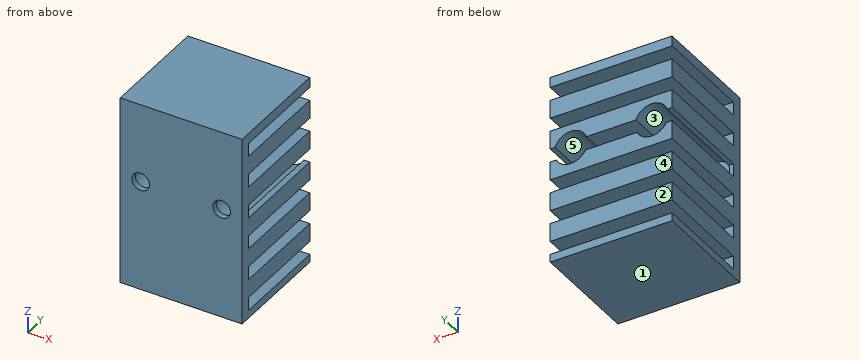
```python
from build123d import *

# Parameters (mm, degrees)
SKETCH1_W           = 11
SKETCH1_H           = 17.14
SKETCH1_R           = 0.8
BOSS_EXTRUDE1_DEPTH = 10
SKETCH3_W           = 1.2
SKETCH3_H           = 9.077755084
CUT_EXTRUDE1_DEPTH  = 18.159396843
SKETCH4_R           = 1.5
CUT_EXTRUDE2_DEPTH  = 9.5


with BuildPart() as part:
    # Sketch1 → Boss-Extrude1 (new body)
    with BuildSketch(Plane(origin=(0, 0, 0), x_dir=(1, 0, 0), z_dir=(0, 1, 0))):
        Rectangle(SKETCH1_W, SKETCH1_H)
        with Locations(Location((3.65, -1.43, 0), (0, 0, 270))):
            Circle(SKETCH1_R, mode=Mode.SUBTRACT)
        with Locations(Location((-3.65, -1.43, 0), (0, 0, 270))):
            Circle(SKETCH1_R, mode=Mode.SUBTRACT)
    extrude(amount=BOSS_EXTRUDE1_DEPTH)

    # Sketch3 → Cut-Extrude1 (cut, through all)
    with BuildSketch(Plane(origin=(5.5, 0, 0), x_dir=(0, 0, -1), z_dir=(1, 0, 0))):
        with Locations((-4.19, 5.461122458)):
            Rectangle(SKETCH3_W, SKETCH3_H)
        with Locations((-7.05, 5.461122458)):
            Rectangle(SKETCH3_W, SKETCH3_H)
        with Locations((-1.33, 5.461122458)):
            Rectangle(SKETCH3_W, SKETCH3_H)
        with Locations((1.53, 5.461122458)):
            Rectangle(SKETCH3_W, SKETCH3_H)
        with Locations((4.39, 5.461122458)):
            Rectangle(SKETCH3_W, SKETCH3_H)
        with Locations((7.25, 5.461122458)):
            Rectangle(SKETCH3_W, SKETCH3_H)
    extrude(amount=-CUT_EXTRUDE1_DEPTH, mode=Mode.SUBTRACT)

    # Sketch4 → Cut-Extrude2 (cut)
    with BuildSketch(Plane(origin=(0, 10, 0), x_dir=(1, 0, 0), z_dir=(0, 1, 0))):
        with Locations(Location((-3.65, -1.43, 0), (0, 0, 270))):
            Circle(SKETCH4_R)
        with Locations(Location((3.65, -1.43, 0), (0, 0, 270))):
            Circle(SKETCH4_R)
    extrude(amount=-CUT_EXTRUDE2_DEPTH, mode=Mode.SUBTRACT)


solid = part.part
```
Check sheet for the modelled part. Datum: model origin and axes. Units: mm. Face numbers are marked on the shaded views. A direction names the side the tool comes from. Give positions to 0.01 mm unless a question says otherwise; leave off trailing zeros. Loops run counter-clockwise (first coordinate to the right, second up) from the corner with the lowest first, then second, coordinate; pieces in that order, holes last. Notation, with made-up numbers: M 58,89 L 114,89 A21 cw 114,95 Z; hole C 6,60 d6. An arc over 180 degrees is marked long. Answer as CSV lines item,"result".
Item 1: Sectioned sample at D-D, the plane z = -7. Enter the section's corners in (x, y).
Reply:
outline,"M -5.5,0 L 5.5,0 L 5.5,0.92 L -5.5,0.92 Z"
Item 2: Sectioned sample at C-C, the plane y = 6.25. State how many separate pieces and enclosed holes the cut face has, then the cut area to 3 significant figures.
Reply:
separate pieces,"7"
enclosed holes,"0"
area,"102 mm^2"
Item 3: Depth check by flat-ended pin: pin 1 Ø0.9 at (x, z) = (-3, 2) entering from +Y; pin 2 Ø1 at (x, z) = (-0.5, 1.5) entering from +Y; pin 3 Ø0.6 at (x, z) = (-5.5, 1.5) entering from +Y. Enter the tip coordinate at first touch or a pass-through.
Reply:
pin 1,"y = 0.5"
pin 2,"y = 10"
pin 3,"y = 0.92"
Item 4: Scan lines: L1, parallel to Z at x = 3.65, y = 0.2; L2, parallel to Y at x = -2.5, z = -4; L3, parallel to X at y = 2, z = 2.25. Record each from-to range of solid material in increasing order.
Reply:
L1,"-8.57 to 0.63, 2.23 to 8.57"
L2,"0 to 0.92"
L3,"-5.5 to -4.91, -2.39 to 2.39, 4.91 to 5.5"
Item 5: Draft check along Z on the marked faces 1, 2 and 3. Enter one of: pulls with the +Z half, pulls with the -Z half, needs draft (parallel to the pull), parting line crosses it, or undercut.
Reply:
face 1,"pulls with the -Z half"
face 2,"needs draft"
face 3,"undercut"
Item 6: Sectioned sample at A-A, the plane z = 1.43. Enter the section's corners in (x, y), then the cut area to 3 significant figures.
Reply:
outline,"M -5.5,0 L -4.45,0 L -4.45,0.5 L -5.15,0.5 L -5.15,0.92 L -5.5,0.92 Z; M -2.85,0 L 2.85,0 L 2.85,0.5 L 2.15,0.5 L 2.15,0.92 L -2.15,0.92 L -2.15,0.5 L -2.85,0.5 Z; M 4.45,0 L 5.5,0 L 5.5,0.92 L 5.15,0.92 L 5.15,0.5 L 4.45,0.5 Z"
area,"6.01 mm^2"
Item 7: Set-up check for the marked faces 4 and 5: record each of +Z, -Z, +X, -X, +Y, -Y from which the full face is reachable in a straight line by a thin tool's end or side.
Reply:
face 4,"+Z, -Z, +X, -X, +Y"
face 5,"+Y"
